from build123d import *

# Parameters (mm, degrees)
SKETCH1_R           = 30
BOSS_EXTRUDE1_DEPTH = 20
SKETCH2_R           = 15
BOSS_EXTRUDE2_DEPTH = 55
SKETCH3_R           = 28
BOSS_EXTRUDE3_DEPTH = 55


with BuildPart() as part:
    # Sketch1 → Boss-Extrude1 (new body)
    with BuildSketch(Plane(origin=(0, 0, 0), x_dir=(0, 0, -1), z_dir=(1, 0, 0))):
        with BuildLine():
            Line((0, -44), (-131, -44))
            ThreePointArc((-131, -44), (-210.210724185, -17.839417698), (-258.260566126, 50.350959788))
            ThreePointArc((-258.260566126, 50.350959788), (-263.903546034, 93.404049189), (-230.531495232, 121.183861184))
            Line((-230.531495232, 121.183861184), (-170.294790462, 242))
            ThreePointArc((-170.294790462, 242), (-179.048984689, 270.890098256), (-171.821418425, 300.199413834))
            ThreePointArc((-171.821418425, 300.199413834), (-138.941281444, 310.421078117), (-127.038840466, 278.111362436))
            Line((-127.038840466, 278.111362436), (-191.024673217, 129.537921032))
            Line((-191.024673217, 129.537921032), (-178.070389074, 92.752237372))
            ThreePointArc((-178.070389074, 92.752237372), (-151.398741624, 57.421955924), (-109.215135044, 44))
            Line((-109.215135044, 44), (0, 44))
            ThreePointArc((0, 44), (44, 0), (0, -44))
        make_face()
        Circle(SKETCH1_R, mode=Mode.SUBTRACT)
    extrude(amount=BOSS_EXTRUDE1_DEPTH)


with BuildPart() as body_2:
    # Mirror2: mirrored copy
    add(part.part.mirror(Plane(origin=(-55, 0, 0), x_dir=(0, 0, 1), z_dir=(1, 0, 0))))


with BuildPart() as part_1:
    add(part.part)

    add(body_2.part)  # Boss-Extrude2 merges body 2
    # Sketch2 → Boss-Extrude2 (add, symmetric)
    with BuildSketch(Plane(origin=(-55, 0, 0), x_dir=(0, 0, -1), z_dir=(1, 0, 0))):
        with Locations(Location((-150, 288, 0), (0, 0, 180))):
            Circle(SKETCH2_R)
    extrude(amount=BOSS_EXTRUDE2_DEPTH, both=True)

    # Sketch3 → Boss-Extrude3 (add, symmetric)
    with BuildSketch(Plane(origin=(-55, 0, 0), x_dir=(0, 0, -1), z_dir=(1, 0, 0))):
        with Locations(Location((-220, 79, 0), (0, 0, 180))):
            Circle(SKETCH3_R)
    extrude(amount=BOSS_EXTRUDE3_DEPTH, both=True)


solid = part_1.part
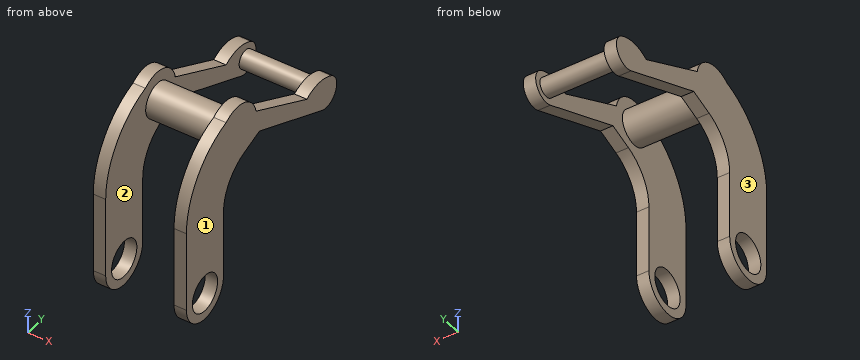
Work out the finished part from the listing and answer in its coordinate system (mm). Face numbers are marked on the shaded views. Round coordinates to 2 decimals unless told otherwise and drop trailing zeros. Write each loop counter-clockwise with the first axis right and the second up, starting at its lowest first coordinate (ties: lowest second). Pieces come first, ordered by that corner, then holes. Notation, with made-up numbers: (-20.5, -26) -> (34.5, -26) arc R24 ccw to (34.5, -10) -> close; hole circle Ø2 at (-29, 25). An arc over 180 degrees is marked (long way). Write each question's results on one line, items separated by ' | '.
Item 1: A cutting plane is placed at B-B, the plane x = -114. Determine the outline of the cut face in (y, z).
Result set:
outline: (-44, 0) arc R44 ccw to (44, 0) -> (44, 109.22) arc R73 cw to (92.75, 178.07) -> (129.54, 191.02) -> (278.11, 127.04) arc R25 ccw to (300.2, 171.82) arc R57 ccw to (242, 170.29) -> (121.18, 230.53) arc R45 ccw to (50.35, 258.26) arc R133 ccw to (-44, 131) -> close; hole circle Ø60 at (0, 0)
Item 2: A cutting plane is placed at D-D, the plane z = 150. Determine the outline of the cut face in (x, y).
Result set:
outline: (-130, -42.64) -> (-110, -42.64) -> (-110, 56.46) -> (-130, 56.46) -> close; (-130, 224.8) -> (-110, 224.8) -> (-110, 273) -> (0, 273) -> (0, 224.8) -> (20, 224.8) -> (20, 313) -> (0, 313) -> (0, 303) -> (-110, 303) -> (-110, 313) -> (-130, 313) -> close; (0, -42.64) -> (20, -42.64) -> (20, 56.46) -> (0, 56.46) -> close
Item 3: Find the intervals of material crossed by line 1 along X through (y, z) = (145.5, 193); line 2 along Y through (x, z) = (4, 90); line 3 along Y through (x, z) = (-120, 120.5), in increasing order. Write a range as [from, to].
Result set:
line 1: [-130, -110], [0, 20] | line 2: [-44, 44] | line 3: [-44, 44.88]
Item 4: A cutting plane is placed at A-A, the plane y = 262. Determine the outline of the cut face in (x, z), plus the area to 3 significant figures.
Result set:
outline: (-130, 133.98) -> (-110, 133.98) -> (-110, 178.11) -> (-130, 178.11) -> close; (0, 133.98) -> (20, 133.98) -> (20, 178.11) -> (0, 178.11) -> close | area: 1,770 mm^2
Item 5: A cutting plane is placed at C-C, the plane y = 0. Determine the outline of the cut face in (x, z), plus the area to 3 significant figures.
Result set:
outline: (-130, -44) -> (-110, -44) -> (-110, -30) -> (-130, -30) -> close; (-130, 30) -> (-110, 30) -> (-110, 229.83) -> (-130, 229.83) -> close; (0, -44) -> (20, -44) -> (20, -30) -> (0, -30) -> close; (0, 30) -> (20, 30) -> (20, 229.83) -> (0, 229.83) -> close | area: 8,550 mm^2
Item 6: Flat-ended cylindrical pins translate along their axes: P1, Ø6, axis at x = -102, z = 136.5, coming from the -Y side; P2, Ø8, axis at x = -5.5, y = 108.5, coming from the +Z side; P3, Ø2, axis at x = -110.5, z = 127.5, coming from the +Y side; P4, Ø10, axis at x = -84.5, z = 186, coming from the +Y side. Find the tip coordinate at first contact, or state that the pin passes through.
Result set:
P1: y = 277.29 | P2: z = 231.57 | P3: y = 300.76 | P4: through
Item 7: The mould has two halves that part along X. Classify the marked faces 1, 2 and 3: +X half, -X half, draft (parallel to the pull), parting line (faces both ways), or undercut.
Result set:
face 1: +X half | face 2: undercut | face 3: -X half
